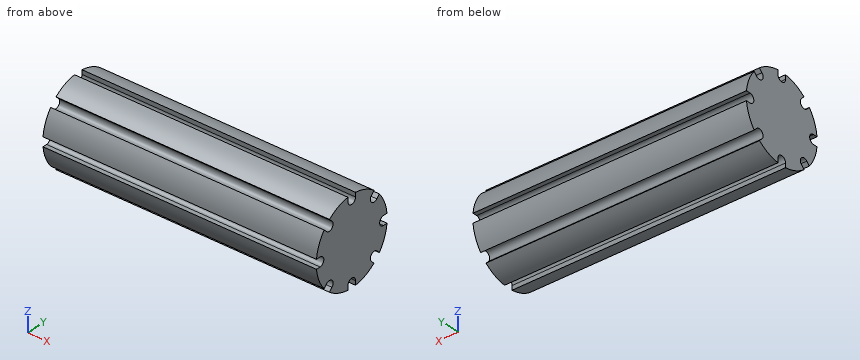
```python
from build123d import *

# Parameters (mm, degrees)
SKETCH_1_R               = 23.5
EXTRUDE_1_DEPTH          = 75
CUT_EXTRUDE_1_DEPTH      = 154.637560512
PATTERN_CIRCULAR_2_COUNT = 8


with BuildPart() as part:
    # 草图1 → 凸台-拉伸1 (new, symmetric)
    with BuildSketch(Plane(origin=(0, 0, 0), x_dir=(0, 0, -1), z_dir=(1, 0, 0))):
        Circle(SKETCH_1_R)
    extrude(amount=EXTRUDE_1_DEPTH, both=True)

    # 草图2 → 切除-拉伸1 (cut, through all)
    with BuildSketch(Plane(origin=(75, 0, 0), x_dir=(0, 0, -1), z_dir=(1, 0, 0))):
        with BuildLine():
            ThreePointArc((-2.5, 21), (0, 18.5), (2.5, 21))
            ThreePointArc((2.5, 21), (1.767766953, 22.767766953), (0, 23.5))
            ThreePointArc((0, 23.5), (-1.251777149, 23.46663704), (-2.5, 23.366642891))
            Line((-2.5, 23.366642891), (-2.5, 21))
        make_face()
        with BuildLine():
            ThreePointArc((0, 23.5), (1.767766953, 22.767766953), (2.5, 21))
            Line((2.5, 21), (2.5, 23.366642891))
            ThreePointArc((2.5, 23.366642891), (1.251777149, 23.46663704), (0, 23.5))
        make_face()
    cut_extrude_1 = extrude(amount=-CUT_EXTRUDE_1_DEPTH, mode=Mode.SUBTRACT)

    # 阵列(圆周)2: 切除-拉伸1 ×8 about axis
    pattern_circular_2_axis = Axis((0, 0, 0), (1, 0, 0))
    for i in range(1, PATTERN_CIRCULAR_2_COUNT):
        add(cut_extrude_1.rotate(pattern_circular_2_axis, i * 360 / PATTERN_CIRCULAR_2_COUNT), mode=Mode.SUBTRACT)


solid = part.part
```
Work out the finished part from the listing and answer in its coordinate system (mm). Give positions to 0.01 mm unless a question says otherwise; leave off trailing zeros. Loops run counter-clockwise (first coordinate to the right, second up) from the corner with the lowest first, then second, coordinate; pieces in that order, holes last. Notation, with made-up numbers: (-32, 59.5) -> (18, 59.5) arc R28 ccw to (18, 86.5) -> close; hole circle Ø3 at (39, 68). An arc over 180 degrees is marked (long way). Put each result on its own line as item: value. Start each with the question number.
Item 1: The part is cut by section B-B (y = 0). Give the vertices of the cut face in (x, z).
Item 2: Find the intervals of material crossed by L1, parallel to Z at x = 46, y = 13.5; L2, parallel to Y at x = -52.5, z = 14; L3, parallel to Z at x = 48.5, y = 14.5, in increasing order. Write a range as [from, to].
Item 3: Each of these flat-tipped pins is pushed along its axis until it touches: P1, Ø8, axis at x = 51.5, y = -8.5, coming from the -Z side; P2, Ø1, axis at x = 27, z = -1.5, coming from the -Y side; P3, Ø10, axis at x = -17, y = 9, coming from the -Z side. Where does it stop, or does it pass through?
Answers below:
1. outline: (-75, -18.5) -> (75, -18.5) -> (75, 18.5) -> (-75, 18.5) -> close
2. L1: [-19.24, -17.04], [-12.74, 12.74], [17.04, 19.24]
2. L2: [-18.87, -17.54], [-12.5, 12.5], [17.54, 18.87]
2. L3: [-18.49, -18.04], [-12.37, 12.37], [18.04, 18.49]
3. P1: z = -23.07
3. P2: y = -19.5
3. P3: z = -23.16
